Part model, mm, in its own coordinate system. Face numbers are marked on the shaded views. A direction names the side the tool comes from. Give positions to 0.01 mm unless a question says otherwise; leave off trailing zeros. Write each loop counter-clockwise with the first axis right and the second up, starting at its lowest first coordinate (ties: lowest second). Pieces come first, ordered by that corner, then holes.
Autodesk Fusion 360 part; units mm, degrees
sketch "Sketch1" plane through (0, 0, 0) normal (0, 0, 1) x (1, 0, 0)
  line L0 (0, 0) -> (35, 0)
  line L1 (35, 30) -> (0, 30)
  line L2 (0, 30) -> (0, 0)
  circle A0 centre (35, 15) radius 2.25
  arc A1 (35, 0) -> (35, 30) centre (35, 15) ccw
  line L3 (15, 0) -> (15, 30)
  line L4 (15, 15) -> (0, 30) construction
  line L5 (7.5, 22.5) -> (7.5, 30) construction
  line L6 (7.5, 22.5) -> (0, 22.5) construction
  circle A2 centre (6.5, 23.5) radius 1
  circle A3 centre (8.5, 23.5) radius 1 construction
  circle A4 centre (8.5, 6.5) radius 1
  line L7 (15, 0) -> (0, 15) construction
  line L8 (7.5, 7.5) -> (7.5, 0) construction
  line L9 (7.5, 7.5) -> (15, 7.5) construction
  point P0 (40, 0)
  point P1 (15, 15)
  dimension "d1" = 30
  dimension "d7" = 35
  dimension "d8" = 35
  dimension "d9" = 4.5
  dimension "d14" = 2
  dimension "d36" = 2
extrude "Extrude1" add sketch "Sketch1" along normal blind 5 contours L0 L1 L2 L3 | L0 L1 A1 L3 | A0 | A2 | A4 makes body 1
hole "Hole1" at (8.5, 6.5, 0) at (6.5, 23.5, 0) direction (0, 0, 1) diameter 2 end through all counterbore diameter 2.3 counterbore depth 1 bodies 1 1
sketch "Sketch2" plane through (0, 0, 5) normal (0, 0, 1) x (-1, 0, 0)
  circle A0 centre (-8.5, -6.5) radius 1
  circle A1 centre (-6.5, -23.5) radius 1
  arc A2 (-35, 0) -> (-35, -30) centre (-35, -15) ccw
  line L0 (-35, -30) -> (0, -30)
  line L1 (0, -30) -> (0, 0)
  line L2 (0, 0) -> (-35, 0)
  circle A3 centre (-35, -15) radius 2.25
fillet "Fillet1" radius 2 3 edges at (17.5, 0, 0) (50, 15, 0) (17.5, 30, 0) on bodies 1
ref_plane "WorkPlane1" through (25, 15, 22.5) normal (0, 0, 1) x (1, 0, 0)
mirror "Mirror1" about plane through (25, 15, 22.5) normal (0, 0, 1) of bodies 1 makes body 2
extrude "Extrude2" cut sketch "Sketch2" against normal blind 4 contours A3 bodies 1
sketch "Sketch3" plane through (0, 0, 40) normal (0, 0, -1) x (1, 0, 0)
  circle A0 centre (8.5, -6.5) radius 1
  circle A1 centre (6.5, -23.5) radius 1
  arc A2 (35, -30) -> (35, 0) centre (35, -15) ccw
  line L0 (35, 0) -> (0, 0)
  line L1 (0, 0) -> (0, -30)
  line L2 (0, -30) -> (35, -30)
  line L3 (31.4, -14.9863) -> (24.6174, -26.7346)
  line L4 (35, -15) -> (24.8695, -28.0239) construction
  arc A3 (24.6174, -26.7346) -> (26.1812, -27.951) centre (25.4835, -27.2346) ccw
  line L5 (35.8992, -18.4859) -> (26.1812, -27.951)
  line L6 (31.4, -14.9863) -> (35.8992, -18.4859) construction
  arc A4 (35.8992, -18.4859) -> (31.4, -14.9863) centre (35, -15) ccw
  point P0 (35, -15)
  point P1 (35, -15)
  dimension "d30" = 2
  dimension "d31" = 5.7
  dimension "d32" = 16.5
  dimension "d33" = 7.2
extrude "Extrude3" cut sketch "Sketch3" against normal blind 1.5 contours L3 A3 L5 A4 bodies 2
hidden bodies 2
equation "d1 = breadth"
equation "breadth = 30 mm"
equation "length = 50 mm"
equation "d7 = length - d6"
equation "d8 = d7"
equation "d27 = ( 35 / 2 ) * 1 mm"
equation "d36 = d14"
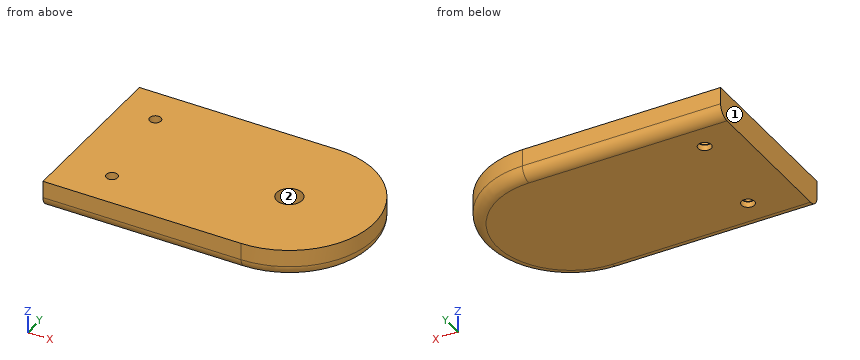
1) Saw through at B-B, the plane z = 2.9. Write the cut outline in (x, y).
Answers follow:
outline: (0, 0) - (35, 0) arc R15 ccw to (35, 30) - (0, 30) - close; hole circle Ø2 at (6.5, 23.5); hole circle Ø2 at (8.5, 6.5); hole circle Ø4.5 at (35, 15)
2) Wall check: L1, parallel to Y at x = 6.5, z = 3.05; L2, parallel to X at y = 15.75, z = 3.5; L3, parallel to Y at x = 8.5, z = 0.5. Give the ranges that are in metal, low to high.
Answers follow:
L1: y = 0 to 22.5, 24.5 to 30
L2: x = 0 to 32.88, 37.12 to 49.98
L3: y = 0.68 to 5.35, 7.65 to 29.32
3) Pin check, flat tips, straight feed: pin 1 Ø1.8 at (x, y) = (8.5, 6) entering from -Z; pin 2 Ø1.2 at (x, y) = (6.5, 23.5) entering from +Z; pin 3 Ø2 at (x, y) = (34, 15) entering from +Z; pin 4 Ø1 at (y, z) = (13.5, 4) entering from +X. Stop position of each tip, or through.
Answers follow:
pin 1: stops at z = 0
pin 2: passes through
pin 3: stops at z = 1
pin 4: stops at x = 49.97
4) 3-axis set-ups, long thin cutter, end or side, ignore diameter. For the marked faces 1 and 2: which of +Z, -Z, +X, -X, +Y, -Y reach the whole face in a straight line?
Answers follow:
face 1: +Z, -Z, -X, +Y, -Y
face 2: +Z
5) Saw through at A-A, the plane x = 8.5. Write the cut outline in (y, z), then the cut area to 3 significant figures.
Answers follow:
outline: (0, 2) arc R2 ccw to (2, 0) - (5.35, 0) - (5.35, 1) - (5.5, 1) - (5.5, 5) - (0, 5) - close; (7.5, 1) - (7.65, 1) - (7.65, 0) - (28, 0) arc R2 ccw to (30, 2) - (30, 5) - (7.5, 5) - close
area: 138 mm2
